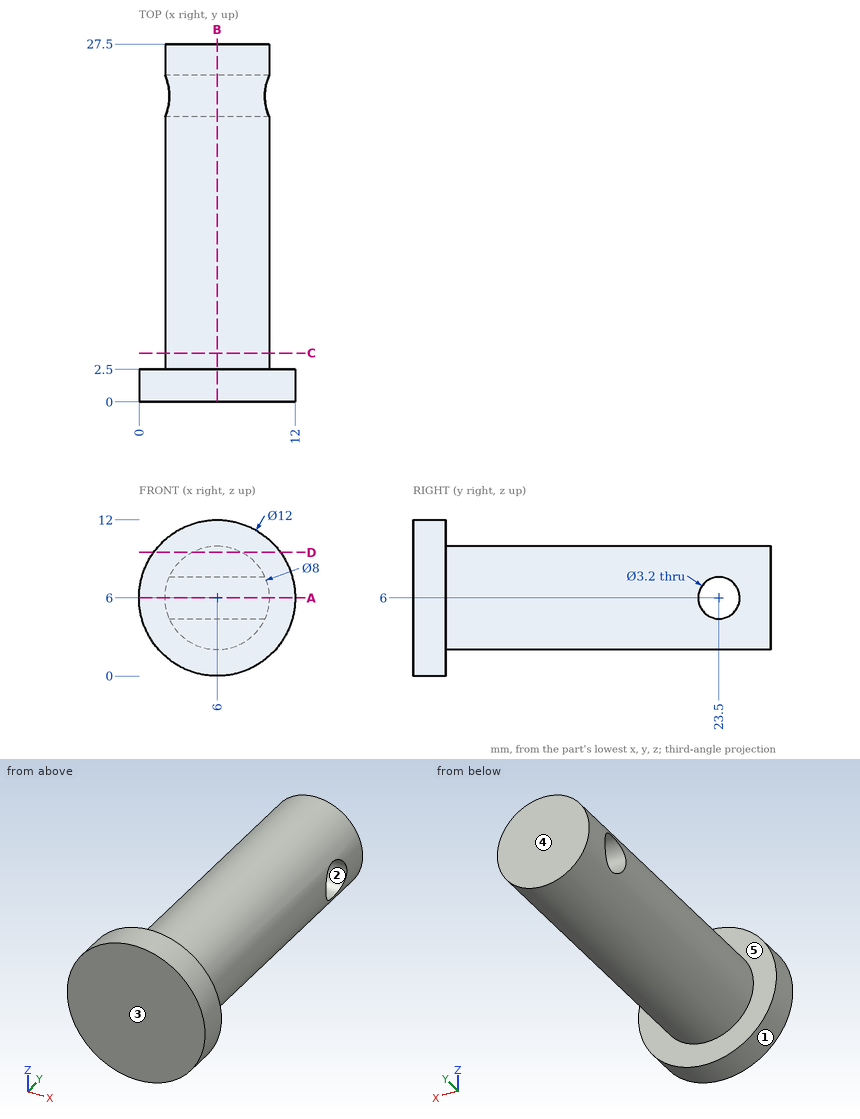
Verification items for this drawing (mm, ordinates from the low corner). A direction names the side the tool comes from. Coordinates: 2 decimals unless noted, no trailing zeros. Write each loop counter-clockwise with the first axis right and the second up, starting at its lowest first coordinate (ties: lowest second). Pieces come first, ordered by that corner, then holes. Notation, with made-up numbers: M -1.5,67.25 L 16.5,67.25 A19 cw 16.5,88.25 Z; hole C 24,84.5 d2. An arc over 180 degrees is marked long. One line per item, written item: value. Start each with the question number.
(1) Tool access check on the marked faces 4 and 5. Record the directions out of +Z, -Z, +X, -X, +Y, -Y that give a thin tool (end or side, any length) a straight path to the whole face; none if there is none.
(2) Release check for a two-part mould opening along Y. For the marked faces 1, 2 and 3 record: released by +Y, released by -Y, zero draft, split by the parting line, or undercut.
(3) Sectioned sample at B-B, the plane x = 6. Enter the section's corners in (y, z).
(4) Sectioned sample at C-C, the plane y = 3.75. Enter the section's corners in (x, z), and give its area (3 significant figures).
(5) Depth check by flat-ended pin: pin 1 (5 mm diameter, centred on y = 9, z = 7.5, fed in from +X); pin 2 (1 mm diameter, centred on y = 7.5, z = 7.5, fed in from +X); pin 3 (2 mm diameter, centred on y = 17, z = 10, fed in from -X). Enter the tip coordinate at first touch or a pass-through.
(6) Scan lines: line 1 along Y through (x, z) = (5.25, 6); line 2 along Y through (x, z) = (7.5, 6.5); line 3 along Y through (x, z) = (3.75, 1.5). Record each from-to range of solid material in increasing order. Write a range as [from, to].
(7) Sectioned sample at D-D, the plane z = 9.5. Enter the section's corners in (x, y), and give its area (3 significant figures).
(8) Sectioned sample at A-A, the plane z = 6. Enter the section's corners in (x, y).
Filled sheet:
1. face 4: +Z, -Z, +X, -X, +Y
1. face 5: +Y
2. face 1: zero draft
2. face 2: undercut
2. face 3: released by -Y
3. outline: M 0,0 L 2.5,0 L 2.5,2 L 27.5,2 L 27.5,10 L 2.5,10 L 2.5,12 L 0,12 Z; hole C 23.5,6 d3.2
4. outline: C 6,6 d8
4. area: 50.3 mm²
5. pin 1: x = 10
5. pin 2: x = 9.87
5. pin 3: x = 3.35
6. line 1: [0, 21.9], [25.1, 27.5]
6. line 2: [0, 21.98], [25.02, 27.5]
6. line 3: [0, 2.5]
7. outline: M 1.13,0 L 10.87,0 L 10.87,2.5 L 7.94,2.5 L 7.94,27.5 L 4.06,27.5 L 4.06,2.5 L 1.13,2.5 Z
7. area: 121 mm²
8. outline: M 0,0 L 12,0 L 12,2.5 L 10,2.5 L 10,21.9 L 2,21.9 L 2,2.5 L 0,2.5 Z; M 2,25.1 L 10,25.1 L 10,27.5 L 2,27.5 Z
